Read the model definition and answer for the solid it produces. Units are mm, in the model's axes. A direction names the side the tool comes from. Round coordinates to 2 decimals unless told otherwise and drop trailing zeros. Answer as a JSON object with one key per item and string values. Group by question number.
Item 1: Consider probe 1 along Z at (x, y) = (0.25, 1.45); probe 2 along X at (y, z) = (-0.2, 1.5); probe 3 along X at (y, z) = (-1.65, 6.5). Determine where each line is inside the solid, lowest interval first. Write a range as from..to.
Item 2: Given P1, Ø2.5, axis at x = 1, y = 0.5, coming from the +Z side; P2, Ø1, axis at x = 1, y = 2, coming from the +Z side; P3, Ø1.5, axis at y = 2, z = 1, coming from the -X side, each flat-ended and moving along its own axis, determine where each tip first touches the part or whether it passes through.
Item 3: The mould has two halves that part along X. Classify faces 3 (the flat face through (0, 0, -3)), 4 (the cylindrical face through (0.525, 0.165, -1.226)): pulls with the +X half, pulls with the -X half, needs draft (parallel to the pull), parting line crosses it, or undercut.
Item 4: For faces 1 (the cylindrical face through (0.525, 0.165, 9.754)), 2 (the cylindrical face through (2.45, -1.01, 1.18)), determine the directions among +Z, -Z, +X, -X, +Y, -Y from which every point of the face is accessible in a straight line to the end or side of a thin tool.
from build123d import *

# Parameters (mm, degrees)
SKETCH003_W = 2.66
SKETCH003_H = 2.25
SKETCH002_W = 2.65
SKETCH002_H = 9
SKETCH001_R = 0.55


with BuildPart() as revolution001:
    # Sketch003 → Revolution001 (revolve)
    with BuildSketch(Plane.XZ):
        with Locations((1.33, 2.975)):
            Rectangle(SKETCH003_W, SKETCH003_H)
    revolve(axis=Axis((0, 0, 0), (0, 0, 1)))


with BuildPart() as revolution:
    # Sketch002 → Revolution (revolve)
    with BuildSketch(Plane.XZ):
        with Locations((1.325, 5)):
            Rectangle(SKETCH002_W, SKETCH002_H)
    revolve(axis=Axis((0, 0, 0), (0, 0, 1)))


with BuildPart() as obj1:
    # Sweep: sweep along a path in Sketch
    with BuildLine(Plane.XZ) as sweep_path:
        Line((0, -3), (0, 10))
        ThreePointArc((0, 10), (0.322183, 10.777817), (1.1, 11.1))
        Line((1.1, 11.1), (3.98, 11.1))
        ThreePointArc((3.98, 11.1), (4.757817, 10.777817), (5.08, 10))
        Line((5.08, 10), (5.08, -3))
    # Sketch001 → Sweep (sweep)
    with BuildSketch(Plane.XY):
        Circle(SKETCH001_R)
    sweep(path=sweep_path.line)

    add(revolution001.part)
    add(revolution.part)


solid = obj1.part
Values found:
{
 "1": {"probe 1": "0.5..9.5", "probe 2": "-2.64..2.64, 4.57..5.59", "probe 3": "-2.07..2.07"},
 "2": {"P1": "z = 11.65", "P2": "z = 9.5", "P3": "x = -2.34"},
 "3": {"face 3": "needs draft", "face 4": "undercut"},
 "4": {"face 1": "none", "face 2": "-Z"}
}
